Verification items for this drawing (mm, ordinates from the low corner). A direction names the side the tool comes from. Round coordinates to 2 decimals unless told otherwise and drop trailing zeros. Write each loop counter-clockwise with the first axis right and the second up, starting at its lowest first coordinate (ties: lowest second). Pieces come first, ordered by that corner, then holes.
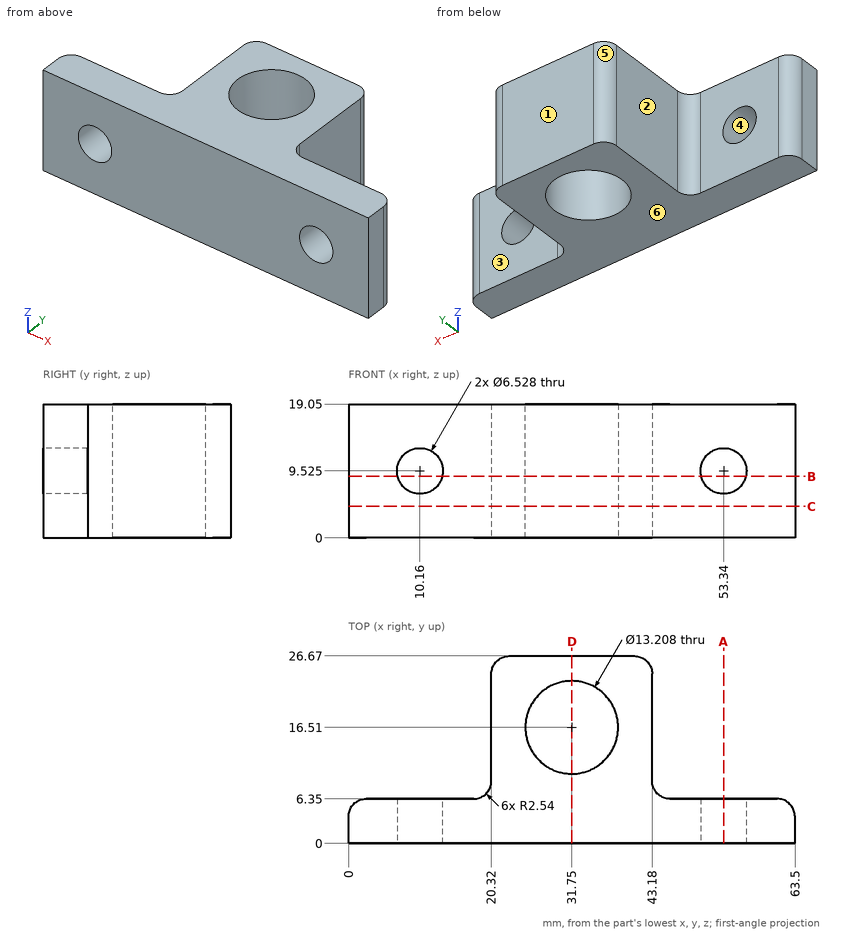
1. Release check for a two-part mould opening along X. For the marked faces 4, 5 and 6 record: +X half, -X half, draft (parallel to the pull), parting line (faces both ways), or undercut.
2. Section check A-A (x = 53.34). Record the cut outline in (y, z), plus the area to 3 significant figures.
3. Scan lines: line 1 along Z through (x, y) = (10.16, 3.5); line 2 along Y through (x, z) = (31.5, 5.5); line 3 along X through (y, z) = (6, 9.75) (1 decimal). Record each from-to range of solid material in increasing order.
4. Access from +Z, -Z, +X, -X, +Y, -Y to the whole of each face (thin tool, end or side, straight path). Record for the marked faces 1, 2 and 3.
5. Section check B-B (z = 8.75). Record the cut outline in (x, y).
6. Section check D-D (x = 31.75). Record the cut outline in (y, z).
7. Depth check by flat-ended pin: pin 1 Ø15 at (x, y) = (31.75, 16.51) entering from -Z; pin 2 Ø4.5 at (x, z) = (56.5, 7.5) entering from +Y; pin 3 Ø4 at (y, z) = (10.5, 8.5) entering from -X; pin 4 Ø4.5 at (y, z) = (18.5, 5) entering from +X. Enter the tip coordinate at first touch or a pass-through.
8. Section check C-C (z = 4.5). Record the cut outline in (x, y), plus the area to 3 significant figures.
Results below:
1. face 4: undercut
1. face 5: -X half
1. face 6: draft
2. outline: (0, 0) - (6.35, 0) - (6.35, 6.26) - (0, 6.26) - close; (0, 12.79) - (6.35, 12.79) - (6.35, 19.05) - (0, 19.05) - close
2. area: 79.5 mm2
3. line 1: z = 0 to 6.26, 12.79 to 19.05
3. line 2: y = 0 to 9.91, 23.11 to 26.67
3. line 3: x = 1.3 to 6.9, 13.4 to 50.1, 56.6 to 62.2
4. face 1: +Z, -Z, +X, -X, +Y
4. face 2: +Z, -Z, -X, +Y
4. face 3: +Z, -Z, +X, +Y
5. outline: (0, 0) - (6.99, 0) - (6.99, 6.35) - (2.54, 6.35) arc R2.54 ccw to (0, 3.81) - close; (13.33, 0) - (50.17, 0) - (50.17, 6.35) - (45.72, 6.35) arc R2.54 cw to (43.18, 8.89) - (43.18, 24.13) arc R2.54 ccw to (40.64, 26.67) - (22.86, 26.67) arc R2.54 ccw to (20.32, 24.13) - (20.32, 8.89) arc R2.54 cw to (17.78, 6.35) - (13.33, 6.35) - close; (56.51, 0) - (63.5, 0) - (63.5, 3.81) arc R2.54 ccw to (60.96, 6.35) - (56.51, 6.35) - close; hole circle Ø13.21 at (31.75, 16.51)
6. outline: (0, 0) - (9.91, 0) - (9.91, 19.05) - (0, 19.05) - close; (23.11, 0) - (26.67, 0) - (26.67, 19.05) - (23.11, 19.05) - close
7. pin 1: stops at z = 0
7. pin 2: stops at y = 6.35
7. pin 3: stops at x = 20.29
7. pin 4: stops at x = 43.18
8. outline: (0, 0) - (63.5, 0) - (63.5, 3.81) arc R2.54 ccw to (60.96, 6.35) - (45.72, 6.35) arc R2.54 cw to (43.18, 8.89) - (43.18, 24.13) arc R2.54 ccw to (40.64, 26.67) - (22.86, 26.67) arc R2.54 ccw to (20.32, 24.13) - (20.32, 8.89) arc R2.54 cw to (17.78, 6.35) - (2.54, 6.35) arc R2.54 ccw to (0, 3.81) - close; hole circle Ø13.21 at (31.75, 16.51)
8. area: 728 mm2
